Here's how the part is built. I have some questions about the finished solid (model axes, mm). A direction names the side the tool comes from. Coordinates: 2 decimals unless noted, no trailing zeros. Write each loop counter-clockwise with the first axis right and the second up, starting at its lowest first coordinate (ties: lowest second). Pieces come first, ordered by that corner, then holes. Notation, with made-up numbers: (89, 87.5) -> (110, 87.5) arc R31 ccw to (110, 124.5) -> close; hole circle Ø2 at (34, 69). An arc over 180 degrees is marked (long way). Put each result on its own line as item: value.
```python
from build123d import *

# Parameters (mm, degrees)
BOSS_EXTRUDE1_DEPTH       = 7.3
SKETCH2_R                 = 2.475
CUT_EXTRUDE1_DEPTH        = 37.841688344
SKETCH3_R                 = 3.125
CUT_EXTRUDE2_DEPTH        = 0.85
LPATTERN1_COUNT           = 5
LPATTERN1_PITCH           = 8
LPATTERN1_COPY_1_SKETCH_R = 3.125
LPATTERN1_COPY_1_DEPTH    = 0.85
LPATTERN1_COPY_2_SKETCH_R = 3.125
LPATTERN1_COPY_2_DEPTH    = 0.85
LPATTERN1_COPY_3_SKETCH_R = 3.125
LPATTERN1_COPY_3_DEPTH    = 0.85
LPATTERN1_COPY_4_SKETCH_R = 3.125
LPATTERN1_COPY_4_DEPTH    = 0.85
CHAMFER1_SIZE             = 0.4


with BuildPart() as part:
    # Sketch1 → Boss-Extrude1 (new body)
    with BuildSketch(Plane(origin=(0, 0, 0), x_dir=(1, 0, 0), z_dir=(0, 1, 0))):
        with BuildLine():
            Line((0, 3.9), (32, 3.9))
            ThreePointArc((32, 3.9), (35.9, 0), (32, -3.9))
            Line((32, -3.9), (0, -3.9))
            ThreePointArc((0, -3.9), (-3.9, 0), (0, 3.9))
        make_face()
    extrude(amount=BOSS_EXTRUDE1_DEPTH)

    # Sketch2 → Cut-Extrude1 (cut, through all)
    with BuildSketch(Plane(origin=(0, 7.3, 0), x_dir=(1, 0, 0), z_dir=(0, 1, 0))):
        with Locations(Location((0, 0, 0), (0, 0, 270))):
            Circle(SKETCH2_R)
    cut_extrude1 = extrude(amount=-CUT_EXTRUDE1_DEPTH, mode=Mode.SUBTRACT)

    # Sketch3 → Cut-Extrude2 (cut)
    with BuildSketch(Plane(origin=(0, 7.3, 0), x_dir=(1, 0, 0), z_dir=(0, 1, 0))):
        with Locations(Location((0, 0, 0), (0, 0, 270))):
            Circle(SKETCH3_R)
    cut_extrude2 = extrude(amount=-CUT_EXTRUDE2_DEPTH, mode=Mode.SUBTRACT)

    # Mirror1: Cut-Extrude2 across plane
    add(cut_extrude2.mirror(Plane.ZX.offset(3.65)), mode=Mode.SUBTRACT)

    # LPattern1: Cut-Extrude1, Cut-Extrude2 ×5
    with Locations(*[(i * LPATTERN1_PITCH, 0, 0) for i in range(1, LPATTERN1_COUNT)]):
        add(cut_extrude1, mode=Mode.SUBTRACT)
        add(cut_extrude2, mode=Mode.SUBTRACT)

    # LPattern1 copy 1 sketch → LPattern1 copy 1 (cut)
    with BuildSketch(Plane(origin=(8, 0, 0), x_dir=(1, 0, 0), z_dir=(0, -1, 0))):
        Circle(LPATTERN1_COPY_1_SKETCH_R)
    extrude(amount=-LPATTERN1_COPY_1_DEPTH, mode=Mode.SUBTRACT)

    # LPattern1 copy 2 sketch → LPattern1 copy 2 (cut)
    with BuildSketch(Plane(origin=(16, 0, 0), x_dir=(1, 0, 0), z_dir=(0, -1, 0))):
        Circle(LPATTERN1_COPY_2_SKETCH_R)
    extrude(amount=-LPATTERN1_COPY_2_DEPTH, mode=Mode.SUBTRACT)

    # LPattern1 copy 3 sketch → LPattern1 copy 3 (cut)
    with BuildSketch(Plane(origin=(24, 0, 0), x_dir=(1, 0, 0), z_dir=(0, -1, 0))):
        Circle(LPATTERN1_COPY_3_SKETCH_R)
    extrude(amount=-LPATTERN1_COPY_3_DEPTH, mode=Mode.SUBTRACT)

    # LPattern1 copy 4 sketch → LPattern1 copy 4 (cut)
    with BuildSketch(Plane(origin=(32, 0, 0), x_dir=(1, 0, 0), z_dir=(0, -1, 0))):
        Circle(LPATTERN1_COPY_4_SKETCH_R)
    extrude(amount=-LPATTERN1_COPY_4_DEPTH, mode=Mode.SUBTRACT)

    # Chamfer1
    # the kernel refuses this chamfer: 0.4 mm, written as the material it takes off along each edge
    with BuildSketch(Plane(origin=(0, 0, 0), x_dir=(0, 0, 1), z_dir=(-1, 0, 0))) as chamfer1_piece_1:
        Polygon((3.125 + CHAMFER1_SIZE, 0), (3.125, CHAMFER1_SIZE), (3.125, 0), align=None)
    revolve(axis=Axis((0, 0, 0), (0, 1, 0)), mode=Mode.SUBTRACT)
    with BuildSketch(Plane(origin=(0, 0, -3.9), x_dir=(0, 0.9996219169112968, -0.027495876610586275), z_dir=(1, 0, 0))) as chamfer1_piece_2:
        Polygon((CHAMFER1_SIZE * 0.999621916911, CHAMFER1_SIZE * 0.0274958766106), (-CHAMFER1_SIZE * 0.0274958766106, CHAMFER1_SIZE * 0.999621916911), (0, 0), align=None)
    extrude(amount=32, mode=Mode.SUBTRACT)
    with BuildSketch(Plane(origin=(32, 0, 0), x_dir=(0, 0, -1), z_dir=(-1, 0, 0))) as chamfer1_piece_3:
        Polygon((3.9, -CHAMFER1_SIZE), (3.9 - CHAMFER1_SIZE, 0), (3.9, 0), align=None)
    revolve(axis=Axis((32, 0, 0), (0, -1, 0)), revolution_arc=180, mode=Mode.SUBTRACT)
    with BuildSketch(Plane(origin=(32, 0, 3.9), x_dir=(0, -0.027495876610586386, -0.9996219169112968), z_dir=(-1, 0, 0))) as chamfer1_piece_4:
        Polygon((CHAMFER1_SIZE * 0.999621916911, -CHAMFER1_SIZE * 0.0274958766106), (-CHAMFER1_SIZE * 0.0274958766106, -CHAMFER1_SIZE * 0.999621916911), (0, 0), align=None)
    extrude(amount=32, mode=Mode.SUBTRACT)
    with BuildSketch(Plane(origin=(0, 0, 0), x_dir=(0, 0, 1), z_dir=(1, 0, 0))) as chamfer1_piece_5:
        Polygon((3.9, -CHAMFER1_SIZE), (3.9 - CHAMFER1_SIZE, 0), (3.9, 0), align=None)
    revolve(axis=Axis((0, 0, 0), (0, -1, 0)), revolution_arc=180, mode=Mode.SUBTRACT)
    with BuildSketch(Plane(origin=(8, 0, 0), x_dir=(1, 0, 0), z_dir=(0, 0, -1))) as chamfer1_piece_6:
        Polygon((3.125 + CHAMFER1_SIZE, 0), (3.125, -CHAMFER1_SIZE), (3.125, 0), align=None)
    revolve(axis=Axis((8, 0, 0), (0, -1, 0)), mode=Mode.SUBTRACT)
    with BuildSketch(Plane(origin=(16, 0, 0), x_dir=(1, 0, 0), z_dir=(0, 0, -1))) as chamfer1_piece_7:
        Polygon((3.125 + CHAMFER1_SIZE, 0), (3.125, -CHAMFER1_SIZE), (3.125, 0), align=None)
    revolve(axis=Axis((16, 0, 0), (0, -1, 0)), mode=Mode.SUBTRACT)
    with BuildSketch(Plane(origin=(24, 0, 0), x_dir=(1, 0, 0), z_dir=(0, 0, -1))) as chamfer1_piece_8:
        Polygon((3.125 + CHAMFER1_SIZE, 0), (3.125, -CHAMFER1_SIZE), (3.125, 0), align=None)
    revolve(axis=Axis((24, 0, 0), (0, -1, 0)), mode=Mode.SUBTRACT)
    with BuildSketch(Plane(origin=(32, 0, 0), x_dir=(1, 0, 0), z_dir=(0, 0, -1))) as chamfer1_piece_9:
        Polygon((3.125 + CHAMFER1_SIZE, 0), (3.125, -CHAMFER1_SIZE), (3.125, 0), align=None)
    revolve(axis=Axis((32, 0, 0), (0, -1, 0)), mode=Mode.SUBTRACT)


solid = part.part
```
Item 1: Please list where these lines run through material, in increasing order: line 1 along X through (y, z) = (7.05, 0) (3 decimals); line 2 along X through (y, z) = (3.8, 0) (3 decimals); line 3 along Z through (x, y) = (32, 0.65) (3 decimals). Write a range as from..to.
Output:
line 1: x = -3.9..-3.125, 3.125..4.875, 11.125..12.875, 19.125..20.875, 27.125..28.875, 35.125..35.9
line 2: x = -3.9..-2.475, 2.475..5.525, 10.475..13.525, 18.475..21.525, 26.475..29.525, 34.475..35.9
line 3: z = -3.9..-3.125, 3.125..3.9
Item 2: Imagine slicing it at B-B on y = 3.5. Write out the boundary of the cut face in (x, z) (3 decimals), then the cut area to 3 significant figures.
Output:
outline: (0, -3.9) -> (32, -3.9) arc R3.9 ccw to (32, 3.9) -> (0, 3.9) arc R3.9 ccw to start; hole circle Ø4.95 at (0, 0); hole circle Ø4.95 at (8, 0); hole circle Ø4.95 at (16, 0); hole circle Ø4.95 at (24, 0); hole circle Ø4.95 at (32, 0)
area: 201 mm²
Item 3: Imagine slicing it at C-C on z = 0.75. State how many separate pieces and enclosed holes the cut face has, then the cut area to 3 significant figures.
Output:
separate pieces: 6
enclosed holes: 0
area: 105 mm²
Item 4: Which directions (+Z, -Z, +X, -X, +Y, -Y) give clear straight access to the entire face, cutting with the end or side of a thin tool? Please do faces 1 (the cylindrical face through (27.1, 6.9, -0.4)), 2 (the cylindrical face through (5.584, 3.689, -0.537)), 3 (the cylindrical face through (13.52, 0.62, -1.9)).
Output:
face 1: +Y
face 2: +Y, -Y
face 3: -Y
Item 5: If we mould it in two halves opening along X, with no side actions, what happens to faces 4 (the conical face through (35.62, 0.12, -0.08)), 5 (the flat face through (30, 0.85, 2)), 6 (the flat face through (16, 4, -3.9))? For each: released by +X, released by -X, zero draft, split by the parting line, or undercut.
Output:
face 4: released by +X
face 5: undercut
face 6: zero draft
Item 6: For P1, Ø1, axis at y = 6, z = -3, coming from the -X side; P2, Ø1.9, axis at x = 9.5, z = -1.5, coming from the -Y side, each with a flat end and sliding along its axis, tell me the tip position at first contact or that it passes through.
Output:
P1: stops at x = -2.99
P2: stops at y = 0.85
